Could you check a few things on this model? Use its own coordinates, in mm. Round coordinates to 2 decimals unless told otherwise and drop trailing zeros. Write each loop counter-clockwise with the first axis right and the second up, starting at its lowest first coordinate (ties: lowest second). Pieces come first, ordered by that corner, then holes. Notation, with made-up numbers: (20, 71.5) -> (32, 71.5) arc R9 ccw to (32, 85.5) -> close; hole circle Ø10 at (19, 45.5). An arc over 180 degrees is marked (long way). Answer as CSV lines item,"result". Start each with the question number.
Q1. Imagine slicing it at C-C on y = 349. Please give me the cut outline in (x, z) (3 decimals).
Q2. Imagine slicing it at A-A on z = 1.1. Please give me the cut outline in (x, y), and give its area (3 significant figures).
Q3. Imagine slicing it at B-B on x = 95. Please give me the cut outline in (y, z) (3 decimals), and give its area (3 significant figures).
Q4. If I drill on line 1 (Y direction, x = 20, z = 0.3); line 2 (Y direction, x = 38, z = 2.05); line 3 (Y direction, x = 145, z = 2.35), over which ranges is the centre line in solid material (lowest first)? Write a range as [from, to].
Q5. Will this pin go through, and if not, where does the flat tip stop? pin 1 Ø1 at (x, z) = (55, 1) entering from +Y.
Autodesk Inventor part; units mm, degrees
ref_plane "YZ Plane" through (0, 0, 0) normal (1, 0, 0) x (0, 1, 0)
ref_plane "XZ Plane" through (0, 0, 0) normal (0, 1, 0) x (-1, 0, 0)
ref_plane "XY Plane" through (0, 0, 0) normal (0, 0, 1) x (1, 0, 0)
sketch "Sketch1" plane through (0, 0, 0) normal (0, 0, 1) x (1, 0, 0)
  line L0 (0, 0) -> (190.5, 0)
  line L1 (190.5, 0) -> (190.5, 635)
  line L2 (190.5, 635) -> (0, 635)
  line L3 (0, 635) -> (0, 0)
  dimension "d0" = 190.5
  dimension "d1" = 635
extrude "Extrusion1" add sketch "Sketch1" along normal blind 3.175
sketch "Sketch2" plane through (0, 0, 3.175) normal (0, 0, 1) x (1, 0, 0)
  line L0 (0, 0) -> (0, 635)
  line L1 (190.5, 0) -> (0, 0)
  line L2 (165.1, 0) -> (0, 0)
  line L3 (0, 177.8) -> (165.1, 0)
  line L4 (0, 635) -> (190.5, 635)
  line L5 (165.1, 635) -> (0, 635)
  line L6 (0, 457.2) -> (165.1, 635)
  line L7 (0, 457.2) -> (0, 635)
  line L8 (165.1, 635) -> (165.1, 0) construction
  line L9 (190.5, 635) -> (190.5, 0)
  dimension "d5" = 177.8
  dimension "d8" = 177.8
  dimension "d9" = 25.4
extrude "Extrusion2" cut sketch "Sketch2" against normal up to next contours L0 L3 L1 | L0 L4 L6
sketch "Sketch4" plane through (0, 0, 3.175) normal (0, 0, 1) x (1, 0, 0)
  line L0 (0, 177.8) -> (0, 457.2)
  line L1 (0, 355.6) -> (50.8, 355.6)
  line L2 (50.8, 355.6) -> (50.8, 279.4)
  line L3 (50.8, 279.4) -> (0, 279.4)
  line L4 (0, 279.4) -> (0, 355.6)
  line L5 (165.1, 635) -> (50.8, 635) construction
  line L6 (50.8, 635) -> (50.8, 355.6) construction
  line L7 (50.8, 279.4) -> (50.8, 0) construction
  line L8 (50.8, 0) -> (165.1, 0) construction
  point P0 (0, 0)
  dimension "d17" = 76.2
  dimension "d18" = 50.8
extrude "Extrusion4" cut sketch "Sketch4" against normal through all
properties part number "Conveyor_Frame_BottomStabilizerPlate" material "Aluminum-6061"
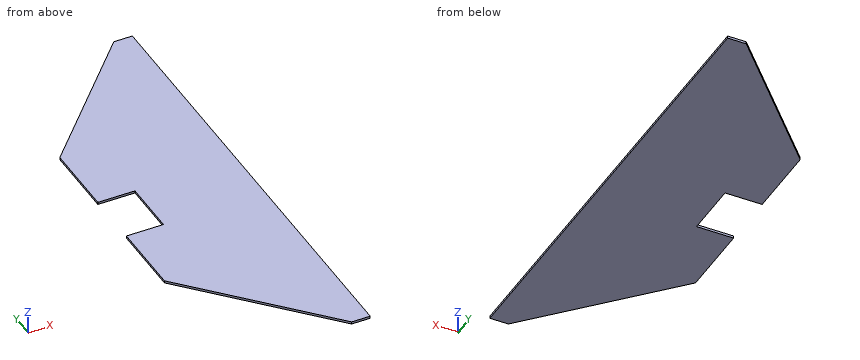
Checks:
1,outline,"(50.8, 0) -> (190.5, 0) -> (190.5, 3.175) -> (50.8, 3.175) -> close"
2,outline,"(0, 177.8) -> (165.1, 0) -> (190.5, 0) -> (190.5, 635) -> (165.1, 635) -> (0, 457.2) -> (0, 355.6) -> (50.8, 355.6) -> (50.8, 279.4) -> (0, 279.4) -> close"
2,area,"87,700 mm^2"
3,outline,"(75.492, 0) -> (559.508, 0) -> (559.508, 3.175) -> (75.492, 3.175) -> close"
3,area,"1,540 mm^2"
4,line 1,"[156.26, 279.4], [355.6, 478.74]"
4,line 2,"[136.88, 279.4], [355.6, 498.12]"
4,line 3,"[21.65, 613.35]"
5,pin 1,"y = 516.97"
